Could you check a few things on this model? Use its own coordinates, in mm. Face numbers are marked on the shaded views. A direction names the side the tool comes from. Give positions to 0.01 mm unless a question says otherwise; leave off trailing zeros. Write each loop counter-clockwise with the first axis right and the second up, starting at its lowest first coordinate (ties: lowest second). Pieces come first, ordered by that corner, then holes. Notation, with made-up numbers: M 53,-20 L 102,-20 A17 ccw 102,11 Z; hole C -16.75,83.5 d8. An arc over 180 degrees is marked long. Use one line per item in the form item = value.
from build123d import *

# Parameters (mm, degrees)
ESQUISSE1_R          = 4
BASE_EXTRUSION_DEPTH = 45
CHANFREIN1_SIZE      = 0.5
ESQUISSE2_R          = 2
BOSS_EXTRU_1_DEPTH   = 4


with BuildPart() as part:
    # Esquisse1 → Base-Extrusion (new body)
    with BuildSketch(Plane.XY):
        Circle(ESQUISSE1_R)
    extrude(amount=BASE_EXTRUSION_DEPTH)

    # Chanfrein1
    chanfrein1_edges = [part.edges().sort_by_distance(p)[0] for p in [
        (-4, 0, 0),
        (-4, 0, 45),
    ]]
    chamfer(chanfrein1_edges, length=CHANFREIN1_SIZE)

    # Esquisse2 → Boss.-Extru.1 (add)
    with BuildSketch(Plane.XY.offset(45)):
        Circle(ESQUISSE2_R)
    extrude(amount=BOSS_EXTRU_1_DEPTH)


solid = part.part
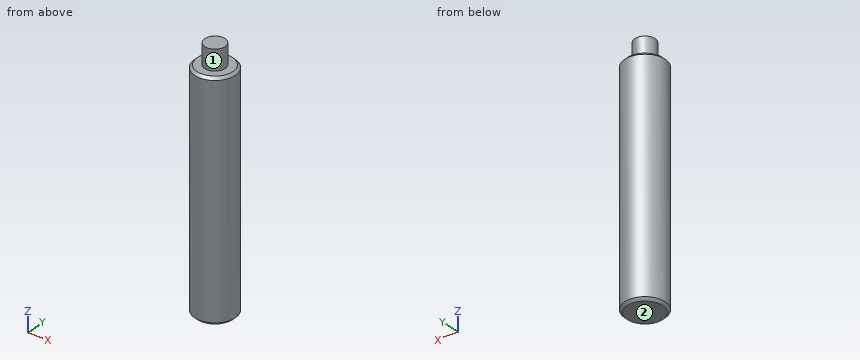
1) For the marked faces 1 and 2, which set-ups out of +Z, -Z, +X, -X, +Y, -Y let a thin tool reach every point of the face, with its end or its side?
Checked values:
face_1 = +Z
face_2 = -Z, +X, -X, +Y, -Y
2) If I drill on L1, parallel to Z at x = -3.5, y = -0.25; L2, parallel to X at y = -0.25, z = 14; L3, parallel to X at y = 3, z = 28, over which ranges is the centre line in solid material (lowest first)?
Checked values:
L1 = 0.01 to 44.99
L2 = -3.99 to 3.99
L3 = -2.65 to 2.65
3) I want a section at A-A, the plane x = 0. Please give me the cut outline in (y, z).
Checked values:
outline = M -4,0.5 L -3.5,0 L 3.5,0 L 4,0.5 L 4,44.5 L 3.5,45 L 2,45 L 2,49 L -2,49 L -2,45 L -3.5,45 L -4,44.5 Z
4) I want a section at D-D, the plane z = 46.5. Please give me the cut outline in (x, y), plus the area to 3 significant figures.
Checked values:
outline = C 0,0 d4
area = 12.6 mm2
5) I want a section at C-C, the plane z = 23.5. Please give me the cut outline in (x, y), plus the area to 3 significant figures.
Checked values:
outline = C 0,0 d8
area = 50.3 mm2
6) For pin 1 Ø4 at (x, z) = (2.5, 6) entering from +Y; pin 2 Ø3 at (y, z) = (-1, 19.5) entering from +X; pin 3 Ø4 at (y, z) = (2.5, 28) entering from -X, each with a flat end and sliding along its axis, tell me the tip position at first contact or that it passes through.
Checked values:
pin_1 = 3.97
pin_2 = 4
pin_3 = -3.97
